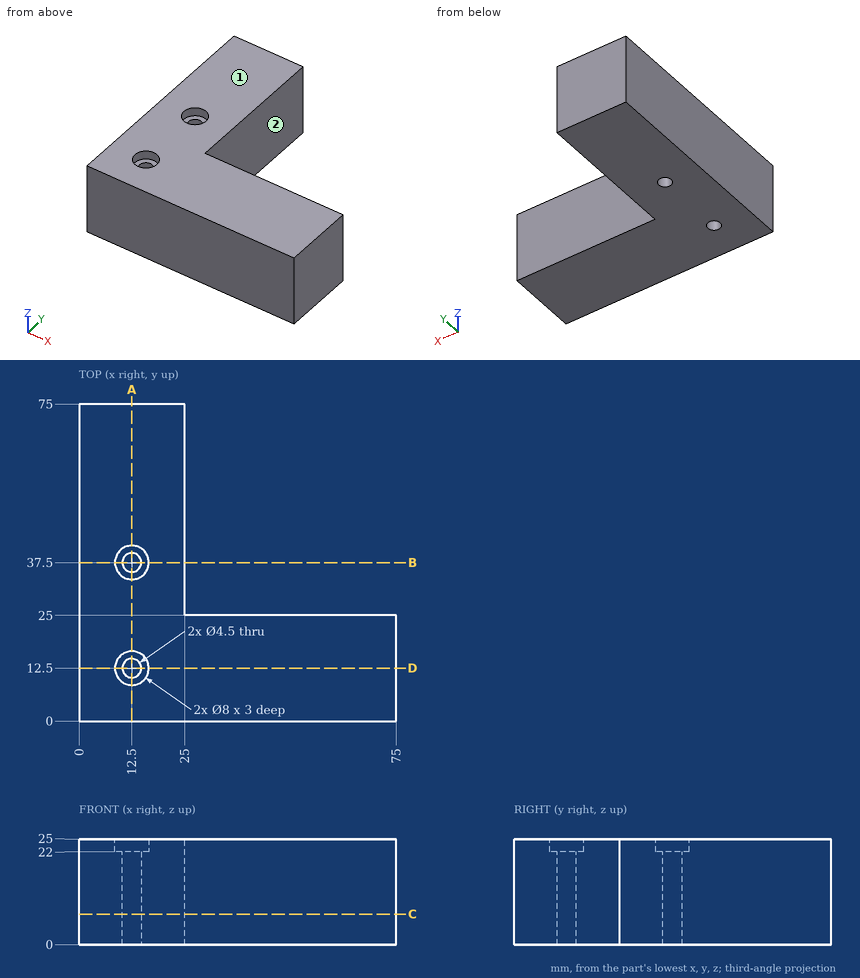
Source: three-view drawing plus pictorial views. Frame: mm from the lowest corner of the part. A direction names the side the tool comes from. Coordinates: 2 decimals unless noted, no trailing zeros. Loops run counter-clockwise (first coordinate to the right, second up) from the corner with the lowest first, then second, coordinate; pieces in that order, holes last. Notation, with made-up numbers: (18.5, 81) - (47.5, 81) arc R33 cw to (47.5, 119) - close; hole circle Ø11 at (8, 25.5). An arc over 180 degrees is marked (long way). One line per item, written item: value. Start each with the question number.
1. Section A-A (x = 12.5). Return the cut outline in (y, z).
2. Section D-D (y = 12.5). Return the cut outline in (x, z), and give its area (3 significant figures).
3. Section C-C (z = 7.25). Return the cut outline in (x, y).
4. Section B-B (y = 37.5). Return the cut outline in (x, z).
5. Set-up query: the marked faces 1 and 2. Return all of +Z, -Z, +X, -X, +Y, -Y with unobstructed straight access to the full face (end or side cutting, diameter ignored); none if empty.
6. Contact query for flat-ended pins moving along their axis: P1, Ø12.5, axis at y = 55.5, z = 8.5, coming from the +X side; P2, Ø12.5, axis at x = 62, z = 13, coming from the +Y side; P3, Ø4, axis at x = 12.5, y = 37.5, coming from the -Z side; P4, Ø4, axis at x = 12.5, y = 11.5, coming from the +Z side. Output: stop coordinate, or through.
7. Ray query, L1, parallel to Y at x = 12.5, z = 23; L2, parallel to Y at x = 12.5, z = 10.5; L3, parallel to Y at x = 64, z = 16.75. Return the intervals inside material, ascending.
Verdict:
1. outline: (0, 0) - (10.25, 0) - (10.25, 22) - (8.5, 22) - (8.5, 25) - (0, 25) - close; (14.75, 0) - (35.25, 0) - (35.25, 22) - (33.5, 22) - (33.5, 25) - (16.5, 25) - (16.5, 22) - (14.75, 22) - close; (39.75, 0) - (75, 0) - (75, 25) - (41.5, 25) - (41.5, 22) - (39.75, 22) - close
2. outline: (0, 0) - (10.25, 0) - (10.25, 22) - (8.5, 22) - (8.5, 25) - (0, 25) - close; (14.75, 0) - (75, 0) - (75, 25) - (16.5, 25) - (16.5, 22) - (14.75, 22) - close
2. area: 1,750 mm2
3. outline: (0, 0) - (75, 0) - (75, 25) - (25, 25) - (25, 75) - (0, 75) - close; hole circle Ø4.5 at (12.5, 12.5); hole circle Ø4.5 at (12.5, 37.5)
4. outline: (0, 0) - (10.25, 0) - (10.25, 22) - (8.5, 22) - (8.5, 25) - (0, 25) - close; (14.75, 0) - (25, 0) - (25, 25) - (16.5, 25) - (16.5, 22) - (14.75, 22) - close
5. face 1: +Z, +X, -X, +Y, -Y
5. face 2: +Z, -Z, +X, +Y
6. P1: stops at x = 25
6. P2: stops at y = 25
6. P3: passes through
6. P4: stops at z = 22
7. L1: y = 0 to 8.5, 16.5 to 33.5, 41.5 to 75
7. L2: y = 0 to 10.25, 14.75 to 35.25, 39.75 to 75
7. L3: y = 0 to 25
